from build123d import *

# Parameters (mm, degrees)
SKETCH_1_R          = 2
EXTRUDE_1_DEPTH     = 2.5
SKETCH_2_W          = 7
SKETCH_2_H          = 12
EXTRUDE_2_DEPTH     = 14
FILLET_1_R          = 2
FILLET_2_R          = 2
FILLET_3_R          = 0.5
CUT_EXTRUDE_1_DEPTH = 0.5
SKETCH_4_R          = 1.5
EXTRUDE_3_DEPTH     = 5
SKETCH_5_R          = 2.5
EXTRUDE_4_DEPTH     = 1


with BuildPart() as part:
    # 草图1 → 凸台-拉伸1 (new body)
    with BuildSketch(Plane(origin=(0, 0, 0), x_dir=(1, 0, 0), z_dir=(0, 1, 0))):
        with BuildLine():
            Line((1, 0), (69, 0))
            ThreePointArc((69, 0), (69.707106781, -0.292893219), (70, -1))
            Line((70, -1), (70, -30))
            ThreePointArc((70, -30), (69.707106781, -30.707106781), (69, -31))
            Line((69, -31), (1, -31))
            ThreePointArc((1, -31), (0.292893219, -30.707106781), (0, -30))
            Line((0, -30), (0, -1))
            ThreePointArc((0, -1), (0.292893219, -0.292893219), (1, 0))
        make_face()
        with Locations(Location((3, -3, 0), (0, 0, 270))):
            Circle(SKETCH_1_R, mode=Mode.SUBTRACT)
        with Locations(Location((67, -3, 0), (0, 0, 90))):
            Circle(SKETCH_1_R, mode=Mode.SUBTRACT)
        with Locations(Location((67, -28, 0), (0, 0, 270))):
            Circle(SKETCH_1_R, mode=Mode.SUBTRACT)
        with Locations(Location((3, -28, 0), (0, 0, 90))):
            Circle(SKETCH_1_R, mode=Mode.SUBTRACT)
    extrude(amount=EXTRUDE_1_DEPTH)

    # 草图2 → 凸台-拉伸2 (add)
    with BuildSketch(Plane(origin=(0, 2.5, 0), x_dir=(1, 0, 0), z_dir=(0, 1, 0))):
        Polygon((61, 0), (9, 0), (9, -9.5), (9, -21.5), (9, -31), (61, -31), (61, -21.5), (61, -9.5), align=None)
        with Locations((5.5, -15.5)):
            Rectangle(SKETCH_2_W, SKETCH_2_H)
        with Locations((64.5, -15.5)):
            Rectangle(SKETCH_2_W, SKETCH_2_H)
    extrude(amount=EXTRUDE_2_DEPTH)

    # 圆角1
    fillet_1_edges = [part.edges().sort_by_distance(p)[0] for p in [
        (9, 9.5, 21.5),
    ]]
    fillet(fillet_1_edges, radius=FILLET_1_R)

    # 圆角2
    fillet_2_edges = [part.edges().sort_by_distance(p)[0] for p in [
        (61, 9.5, 9.5),
        (9, 9.5, 9.5),
        (61, 9.5, 21.5),
    ]]
    fillet(fillet_2_edges, radius=FILLET_2_R)

    # 圆角3
    fillet_3_edges = [part.edges().sort_by_distance(p)[0] for p in [
        (0, 0, 15.5),
        (0.292893219, 0, 0.292893219),
        (35, 0, 0),
        (69.707106781, 0, 0.292893219),
        (61, 16.5, 3.75),
        (61, 9.5, 0),
        (9, 9.5, 0),
        (2, 9.5, 9.5),
        (2, 9.5, 21.5),
        (9, 9.5, 31),
        (61, 9.5, 31),
        (68, 16.5, 15.5),
        (68, 9.5, 21.5),
        (68, 9.5, 9.5),
        (35, 16.5, 0),
        (9, 16.5, 3.75),
        (2, 16.5, 15.5),
        (35, 16.5, 31),
        (9, 16.5, 27.25),
        (4.5, 16.5, 21.5),
        (8.414213562, 16.5, 22.085786438),
        (70, 0, 15.5),
        (65.5, 16.5, 21.5),
        (69.707106781, 0, 30.707106781),
        (61, 16.5, 27.25),
        (65.5, 16.5, 9.5),
        (35, 0, 31),
        (4.5, 16.5, 9.5),
        (61.585786438, 16.5, 22.085786438),
        (0.292893219, 0, 30.707106781),
        (61.585786438, 16.5, 8.914213562),
        (8.414213562, 16.5, 8.914213562),
    ]]
    fillet(fillet_3_edges, radius=FILLET_3_R)

    # 草图3 → 切除-拉伸1 (cut)
    with BuildSketch(Plane.XZ):
        with BuildLine():
            Line((16.290844115, 25.013544626), (32.187512514, 25.013544626))
            ThreePointArc((32.187512514, 25.013544626), (41.70105714, 15.5), (32.187512514, 5.986455374))
            Line((32.187512514, 5.986455374), (16.290844115, 5.986455374))
            ThreePointArc((16.290844115, 5.986455374), (6.777299489, 15.5), (16.290844115, 25.013544626))
        make_face()
    extrude(amount=-CUT_EXTRUDE_1_DEPTH, mode=Mode.SUBTRACT)

    # 草图4 → 凸台-拉伸3 (add)
    with BuildSketch(Plane.ZY.offset(-2)):
        with Locations(Location((15.5, 9.25, 0), (0, 0, 180))):
            Circle(SKETCH_4_R)
    extrude(amount=EXTRUDE_3_DEPTH)

    # 草图5 → 凸台-拉伸4 (add)
    with BuildSketch(Plane.ZY.offset(-2)):
        with Locations(Location((15.5, 9.25, 0), (0, 0, 180))):
            Circle(SKETCH_5_R)
    extrude(amount=EXTRUDE_4_DEPTH)


solid = part.part
Here's how the part is built. I have some questions about the finished solid (model axes, mm). A direction names the side the tool comes from. Coordinates: 2 decimals unless noted, no trailing zeros. Write each loop counter-clockwise with the first axis right and the second up, starting at its lowest first coordinate (ties: lowest second). Pieces come first, ordered by that corner, then holes. Notation, with made-up numbers: (-21, 68) - (8, 68) arc R13 cw to (8, 88) - close; hole circle Ø11 at (13.5, 74). An arc over 180 degrees is marked (long way). Use one line per item in the form item = value.
1) On a 3-axis mill with a long thin cutter (end or side, diameter ignored), from which of +Z, -Z, +X, -X, +Y, -Y can I reach the whole of each face in a straight line? I mean faces 5 (the flat face through (5, 9, 21.5)), 6 (the flat face through (68.5, 2.5, 15.3)), 7 (the flat face through (65, 9, 9.5)), 8 (the cylindrical face through (-1, 9.2, 17)). Say none if no direction works.
Solved:
face_5 = +Z, -X, +Y
face_6 = +X, +Y
face_7 = -Z, +X, +Y
face_8 = -X
2) Thinking about a two-plate mould opening in Y: for faces 1 (the cylindrical face through (1.507, 10.771, 17.484)), 2 (the flat face through (35, 16.5, 15)), 3 (the flat face through (24, 0.5, 16)), 4 (the flat face through (-3, 9, 16)), which applies, released by +Y, released by -Y, zero draft, split by the parting line, or undercut?
Solved:
face_1 = undercut
face_2 = released by +Y
face_3 = released by -Y
face_4 = zero draft
3) Suppose I cut it at A-A, the plane z = 3. Write out the boundary of the cut face in (x, y).
Solved:
outline = (0, 0.5) arc R0.5 ccw to (0.5, 0) - (1, 0) - (1, 2.5) - (0, 2.5) - close; (5, 0) - (65, 0) - (65, 2.5) - (61, 2.5) - (61, 16) arc R0.5 ccw to (60.5, 16.5) - (9.5, 16.5) arc R0.5 ccw to (9, 16) - (9, 2.5) - (5, 2.5) - close; (69, 0) - (69.5, 0) arc R0.5 ccw to (70, 0.5) - (70, 2.5) - (69, 2.5) - close
4) Suppose I cut it at D-D, the plane z = 12. Write out the boundary of the cut face in (x, y).
Solved:
outline = (0, 0.5) arc R0.5 ccw to (0.5, 0) - (7.44, 0) - (7.44, 0.5) - (41.03, 0.5) - (41.03, 0) - (69.5, 0) arc R0.5 ccw to (70, 0.5) - (70, 2.5) - (68, 2.5) - (68, 16) arc R0.5 ccw to (67.5, 16.5) - (2.5, 16.5) arc R0.5 ccw to (2, 16) - (2, 2.5) - (0, 2.5) - close
5) I need wall thicknesses on line 1 (X direction, y = 1.65, z = 28); line 2 (Y direction, x = 8, z = 7); line 3 (Y direction, x = 29, z = 8). Which ranges of each line are inside material? Lowest first, please.
Solved:
line_1 = 0 to 1, 5 to 65, 69 to 70
line_2 = 0 to 2.5
line_3 = 0.5 to 16.5
6) Suppose I cut it at C-C, the plane x = 17.5. Write out the boundary of the cut face in (y, z).
Solved:
outline = (0, 0.5) arc R0.5 ccw to (0.5, 0) - (16, 0) arc R0.5 ccw to (16.5, 0.5) - (16.5, 30.5) arc R0.5 ccw to (16, 31) - (0.5, 31) arc R0.5 ccw to (0, 30.5) - (0, 25.01) - (0.5, 25.01) - (0.5, 5.99) - (0, 5.99) - close
7) I'm going to push flat-ended pins straight in: P1, Ø4.5, axis at x = 67, z = 28, coming from the +Y side; P2, Ø5.5, axis at y = 6.5, z = 3.5, coming from the -X side; P3, Ø1.3, axis at x = 66.5, y = 11, coming from the -Z side. Where does each tip first touch, or does it pass through?
Solved:
P1 = 2.5
P2 = 9
P3 = 9.5
